The listing builds one solid part. Answer for the finished solid, in the listing's coordinates (mm). A direction names the side the tool comes from. Give positions to 0.01 mm unless a question says otherwise; leave off trailing zeros. Write each loop counter-clockwise with the first axis right and the second up, starting at its lowest first coordinate (ties: lowest second). Pieces come first, ordered by that corner, then holes. Notation, with made-up numbers: (-4.75, 57) -> (47.25, 57) arc R16 cw to (47.25, 82) -> close; hole circle Ø9 at (60.5, 40.25). An arc over 180 degrees is marked (long way). One line per question, with ' | ' between items.
from build123d import *

# Parameters (mm, degrees)
ESQUISSE1_W             = 18
ESQUISSE1_H             = 30
BOSS_EXTRU_1_DEPTH      = 70
ESQUISSE2_R             = 4
BOSS_EXTRU_2_DEPTH      = 10
ESQUISSE3_R             = 4
ENL_V_MAT_EXTRU_1_DEPTH = 52
ESQUISSE4_W             = 20
ESQUISSE4_H             = 20
ENL_V_MAT_EXTRU_2_DEPTH = 52


with BuildPart() as part:
    # Esquisse1 → Boss.-Extru.1 (new body)
    with BuildSketch(Plane.XY):
        Rectangle(ESQUISSE1_W, ESQUISSE1_H)
    extrude(amount=BOSS_EXTRU_1_DEPTH)

    # Esquisse2 → Boss.-Extru.2 (add)
    with BuildSketch(Plane(origin=(0, 15, 0), x_dir=(1, 0, 0), z_dir=(0, 1, 0))):
        with Locations((0, -12.75)):
            Circle(ESQUISSE2_R)
    boss_extru_2 = extrude(amount=BOSS_EXTRU_2_DEPTH)

    # Symétrie1: Boss.-Extru.2 across plane
    add(boss_extru_2.mirror(Plane.ZX))

    # Symétrie2: Boss.-Extru.2 across plane
    add(boss_extru_2.mirror(Plane.XY.offset(35)))

    # Esquisse3 → Enlèv. mat.-Extru.1 (cut)
    with BuildSketch(Plane(origin=(0, 25, 0), x_dir=(1, 0, 0), z_dir=(0, 1, 0))):
        with Locations((0, -57.25)):
            Circle(ESQUISSE3_R)
    extrude(amount=-ENL_V_MAT_EXTRU_1_DEPTH, mode=Mode.SUBTRACT)

    # Esquisse4 → Enlèv. mat.-Extru.2 (cut)
    with BuildSketch(Plane(origin=(9, 0, 0), x_dir=(0, 0, -1), z_dir=(1, 0, 0))):
        with Locations((-60, 0)):
            Rectangle(ESQUISSE4_W, ESQUISSE4_H)
    extrude(amount=-ENL_V_MAT_EXTRU_2_DEPTH, mode=Mode.SUBTRACT)


solid = part.part
Item 1: Consider line 1 (Z direction, x = 0, y = -12.9); line 2 (X direction, y = 11.9, z = 57.25); line 3 (Y direction, x = -4.75, z = 57). Determine where each line is inside the solid, lowest interval first. Write a range as [from, to].
Answers below:
line 1: [0, 53.25], [61.25, 70] | line 2: [-9, -4], [4, 9] | line 3: [-15, -10], [10, 15]
Item 2: Find section A-A (z = 57.25). Write down the section's boundary in (x, y), then the cut area to 3 significant figures.
Answers below:
outline: (-9, -15) -> (-4, -15) -> (-4, -10) -> (-9, -10) -> close; (-9, 10) -> (-4, 10) -> (-4, 15) -> (-9, 15) -> close; (4, -15) -> (9, -15) -> (9, -10) -> (4, -10) -> close; (4, 10) -> (9, 10) -> (9, 15) -> (4, 15) -> close | area: 100 mm²
Item 3: A tool of negligible diameter and unlimited length cuts with its end or side. For faces 4 (the face through (-0.867, -19.93, 16.655)), 5 (the face through (0, 10, 62)), 6 (the face through (-0.867, 19.93, 16.655)), 7 (the face through (0, -25, 13)), from which of +Z, -Z, +X, -X, +Y, -Y can it reach the whole face along a straight path? Write none if from no direction.
Answers below:
face 4: -Y | face 5: +Z, +X, -X | face 6: +Y | face 7: +Z, -Z, +X, -X, -Y
Item 4: Find section C-C (z = 12.75). Write down the section's boundary in (x, y).
Answers below:
outline: (-9, -15) -> (-4, -15) -> (-4, -25) -> (4, -25) -> (4, -15) -> (9, -15) -> (9, 15) -> (4, 15) -> (4, 25) -> (-4, 25) -> (-4, 15) -> (-9, 15) -> close
Item 5: Find section D-D (x = -7.5). Write down the section's boundary in (y, z).
Answers below:
outline: (-15, 0) -> (15, 0) -> (15, 70) -> (10, 70) -> (10, 50) -> (-10, 50) -> (-10, 70) -> (-15, 70) -> close
Item 6: Determine the mould class of faces 1 (the face through (0, 25, 13)), 2 (the face through (0, 0, 0)), 3 (the face through (0, -10, 62)) for opening direction Y: pulls with the +Y half, pulls with the -Y half, needs draft (parallel to the pull), parting line crosses it, or undercut.
Answers below:
face 1: pulls with the +Y half | face 2: needs draft | face 3: undercut
Item 7: Flat-ended cylindrical pins translate along their axes: pin 1 (1 mm diameter, centred on x = 0.5, z = 48.5, fed in from +Y); pin 2 (5.5 mm diameter, centred on x = -1, z = 59.5, fed in from -Y). Find the tip coordinate at first contact, or state that the pin passes through.
Answers below:
pin 1: y = 15 | pin 2: y = -15
Item 8: Find section B-B (x = 2.75). Write down the section's boundary in (y, z), then the cut area to 3 significant figures.
Answers below:
outline: (-25, 9.85) -> (-15, 9.85) -> (-15, 0) -> (15, 0) -> (15, 9.85) -> (25, 9.85) -> (25, 15.65) -> (15, 15.65) -> (15, 54.35) -> (10, 54.35) -> (10, 50) -> (-10, 50) -> (-10, 54.35) -> (-15, 54.35) -> (-15, 15.65) -> (-25, 15.65) -> close; (-15, 60.15) -> (-10, 60.15) -> (-10, 70) -> (-15, 70) -> close; (10, 60.15) -> (15, 60.15) -> (15, 70) -> (10, 70) -> close | area: 1,760 mm²
